from build123d import *

# Parameters (mm, degrees)
BOSS_EXTRUDE1_DEPTH = 1603
CUT_EXTRUDE1_DEPTH  = 1187.25


with BuildPart() as part:
    # Sketch2 → Boss-Extrude1 (new body)
    with BuildSketch(Plane(origin=(0, 0, 0), x_dir=(1, 0, 0), z_dir=(0, 1, 0))):
        Polygon((577.35026919, 0), (288.675134595, 500), (-288.675134595, 500), (-577.35026919, 0), (-288.675134595, -500), (288.675134595, -500), align=None)
    extrude(amount=BOSS_EXTRUDE1_DEPTH)

    # Sketch3 → Cut-Extrude1 (cut)
    with BuildSketch(Plane(origin=(0, 400.75, 0), x_dir=(1, 0, 0), z_dir=(0, 1, 0))):
        Polygon((575.040868113, 0), (287.520434056, 498), (-287.520434056, 498), (-575.040868113, 0), (-287.520434056, -498), (287.520434056, -498), align=None)
    extrude(amount=CUT_EXTRUDE1_DEPTH, mode=Mode.SUBTRACT)


solid = part.part
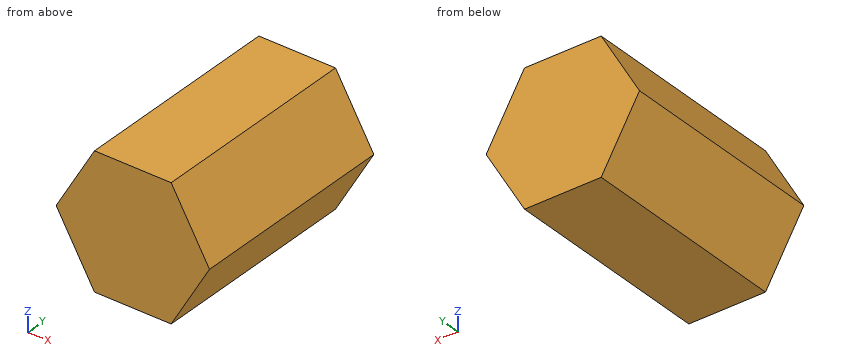
Model file for the job. Use its own axes, mm. Give positions to 0.01 mm unless a question says otherwise; leave off trailing zeros. Loops run counter-clockwise (first coordinate to the right, second up) from the corner with the lowest first, then second, coordinate; pieces in that order, holes last.
1) Saw through at A-A (y = 485). Write the cut outline in (x, z).
2) Saw through at B-B (z = 25). Write the cut outline in (x, y).
3) Flat gauge pins, fed straight in: pin 1 Ø10 at (y, z) = (1052, 229) entering from +X; pin 2 Ø1 at (y, z) = (632, 112.5) entering from -X; pin 3 Ø12 at (x, y) = (-382, 712.5) entering from +Z. Where does each tip first touch, or does it go through?
4) Wall check: line 1 (Z direction, x = -67, y = 805); line 2 (Y direction, x = -148.5, z = 450.5); line 3 (Z direction, x = 437, y = 1032.5). Give the ranges that are in metal, low to high.
5) Saw through at C-C (x = 76). Write the cut outline in (y, z), plus the area to 4 significant figures.
Answer block:
1. outline: (-577.35, 0) - (-288.68, -500) - (288.68, -500) - (577.35, 0) - (288.68, 500) - (-288.68, 500) - close; hole (-575.04, 0) - (-287.52, -498) - (287.52, -498) - (575.04, 0) - (287.52, 498) - (-287.52, 498) - close
2. outline: (-562.92, 0) - (562.92, 0) - (562.92, 1603) - (-562.92, 1603) - close; hole (-560.61, 400.75) - (560.61, 400.75) - (560.61, 1588) - (-560.61, 1588) - close
3. pin 1: stops at x = 448.02
3. pin 2: stops at x = -512.69
3. pin 3: stops at z = 348.75
4. line 1: z = -500 to -498, 498 to 500
4. line 2: y = 0 to 400.75, 1588 to 1603
4. line 3: z = -243.09 to -239.09, 239.09 to 243.09
5. outline: (0, -500) - (1603, -500) - (1603, 500) - (0, 500) - close; hole (400.75, -498) - (1588, -498) - (1588, 498) - (400.75, 498) - close
5. area: 420,500 mm2
